Source: CAD feature listing. Evaluate the final solid. Frame: model axes, mm. A direction names the side the tool comes from. Coordinates: 2 decimals unless noted, no trailing zeros. Order: outer loops, then holes, each group sorted by start corner. A loop starts at its lowest first (then second) coordinate and runs counter-clockwise, first axis right, second up.
```python
from build123d import *

# Parameters (mm, degrees)
CROQUIS1_W              = 200
CROQUIS1_H              = 100
SALIENTE_EXTRUIR1_DEPTH = 200
CORTAR_EXTRUIR1_DEPTH   = 200
CORTAR_EXTRUIR2_DEPTH   = 200
VACIADO1_T              = 4


with BuildPart() as part:
    # Croquis1 → Saliente-Extruir1 (new body)
    with BuildSketch(Plane.XY):
        Rectangle(CROQUIS1_W, CROQUIS1_H)
    extrude(amount=SALIENTE_EXTRUIR1_DEPTH)

    # Croquis18 → Cortar-Extruir1 (cut)
    with BuildSketch(Plane.ZY.offset(100)):
        Polygon((0, 50), (200, 50), (200, 25), align=None)
    extrude(amount=-CORTAR_EXTRUIR1_DEPTH, mode=Mode.SUBTRACT)

    # Croquis20 → Cortar-Extruir2 (cut)
    with BuildSketch(Plane.ZY.offset(100)):
        Polygon((0, -50), (200, -50), (200, -25), align=None)
    extrude(amount=-CORTAR_EXTRUIR2_DEPTH, mode=Mode.SUBTRACT)

    # Vaciado1 (no face opened: a closed hollow body)
    add(offset(amount=-VACIADO1_T, mode=Mode.PRIVATE), mode=Mode.SUBTRACT)


solid = part.part
```
1. Section query B-B on z = 85. Return loops of the section in (x, y) (3 decimals).
Findings:
outline: (-100, -39.375) - (100, -39.375) - (100, 39.375) - (-100, 39.375) - close; hole (-96, -35.344) - (96, -35.344) - (96, 35.344) - (-96, 35.344) - close
2. Ray query, line 1 (Z direction, x = -10.5, y = -14); line 2 (X direction, y = -19, z = 100.5); line 3 (Y direction, x = -5, z = 148). Return the intervals inside material, ascending.
Findings:
line 1: z = 0 to 4, 196 to 200
line 2: x = -100 to -96, 96 to 100
line 3: y = -31.5 to -27.47, 27.47 to 31.5
3. Section query A-A on x = -59.5. Return loops of the section in (y, z), plus the area to 3 significant figures.
Findings:
outline: (-50, 0) - (50, 0) - (25, 200) - (-25, 200) - close; hole (-45.47, 4) - (45.47, 4) - (21.47, 196) - (-21.47, 196) - close
area: 2,150 mm2
4. Pin query (flat end, axial travel): P1, Ø8, axis at x = 76, z = 73.5, coming from the -Y side; P2, Ø4, axis at x = -15, z = 146.5, coming from the +Y side; P3, Ø1.5, axis at x = 5.5, z = 124, coming from the -Y side. Return the tip coordinate at first contact, or that it passes through.
Findings:
P1: stops at y = -41.31
P2: stops at y = 31.94
P3: stops at y = -34.59
5. Draft query along Z for faces 3 (the face through (-100, -1, 76)), 4 (the face through (96, -1, 77)), 5 (the face through (-1, 1, 0)), 6 (the face through (-1.4, -37.325, 101.4)). Return one class per face: released by +Z, released by -Z, zero draft, split by the parting line, or undercut.
Findings:
face 3: zero draft
face 4: undercut
face 5: released by -Z
face 6: released by +Z
6. Access query for faces 1 (the face through (-1.34, -33.3, 101.34)), 2 (the face through (100, -1, 76)). Directions: +Z, -Z, +X, -X, +Y, -Y. A direction counts if a zero-diameter tool reaches every point of the face in a straight line with its end or side. Return the directions, or none.
Findings:
face 1: none
face 2: +Z, -Z, +X, +Y, -Y
